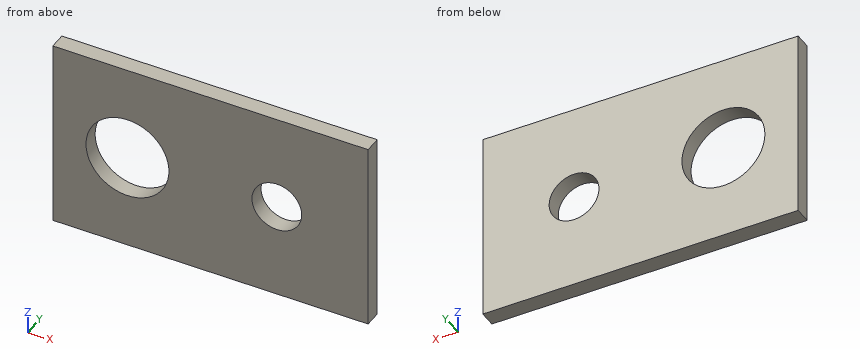
```python
from build123d import *

# Parameters (mm, degrees)
F0_W     = 60.325
F0_H     = 36.5125
F1_DEPTH = 3.175
F3_D     = 15.875
F5_D     = 9.525


with BuildPart() as f1:
    # F0 (on Front) → F1 (new body)
    with BuildSketch(Plane.XZ):
        Rectangle(F0_W, F0_H)
    extrude(amount=F1_DEPTH)

    # F3 (through all)
    with Locations(Plane.XZ.offset(3.175)):
        with Locations((-15.875, 0)):
            Hole(F3_D / 2)

    # F5 (through all)
    with Locations(Plane.XZ.offset(3.175)):
        with Locations((12.7, 0)):
            Hole(F5_D / 2)


solid = f1.part
```
Source: CAD feature listing. Evaluate the final solid. Frame: model axes, mm. Give positions to 0.01 mm unless a question says otherwise; leave off trailing zeros. Loops run counter-clockwise (first coordinate to the right, second up) from the corner with the lowest first, then second, coordinate; pieces in that order, holes last. Notation, with made-up numbers: (43.5, 89.5) -> (100.5, 89.5) arc R31 ccw to (100.5, 114.5) -> close; hole circle Ø6 at (-28, -34). An arc over 180 degrees is marked (long way). Use a Markdown table: item, result. Add a question column.
(1) Section query A-A (z = 0). Output: boundary loops of the cut face in (x, y) (1 decimal).
(2) Section query B-B (x = 12.7). Output: boundary loops of the cut face in (y, z) (1 decimal).
(3) First-contact query: pin 1 Ø9.5 at (x, z) = (-15.875, 0) entering from +Y. Flat tip, straight axial feed; report the tip coordinate or a pass-through.
(4) Ray query, line 1 (Z direction, x = 12.7, y = -1); line 2 (X direction, y = -0.9, z = -2.5); line 3 (X direction, y = -1.85, z = 3.5). Return the intervals inside material, ascending.
(5) Section query C-C (y = -1.65). Output: boundary loops of the cut face in (x, z) (1 decimal).
Checked values:
| question | item | result |
|---|---|---|
| 1 | outline | (-30.2, -3.2) -> (-23.8, -3.2) -> (-23.8, 0) -> (-30.2, 0) -> close; (-7.9, -3.2) -> (7.9, -3.2) -> (7.9, 0) -> (-7.9, 0) -> close; (17.5, -3.2) -> (30.2, -3.2) -> (30.2, 0) -> (17.5, 0) -> close |
| 2 | outline | (-3.2, -18.3) -> (0, -18.3) -> (0, -4.8) -> (-3.2, -4.8) -> close; (-3.2, 4.8) -> (0, 4.8) -> (0, 18.3) -> (-3.2, 18.3) -> close |
| 3 | pin 1 | through |
| 4 | line 1 | -18.26 to -4.76, 4.76 to 18.26 |
| 4 | line 2 | -30.16 to -23.41, -8.34 to 8.65, 16.75 to 30.16 |
| 4 | line 3 | -30.16 to -23, -8.75 to 9.47, 15.93 to 30.16 |
| 5 | outline | (-30.2, -18.3) -> (30.2, -18.3) -> (30.2, 18.3) -> (-30.2, 18.3) -> close; hole circle Ø15.9 at (-15.9, 0); hole circle Ø9.5 at (12.7, 0) |
